from build123d import *

# Parameters (mm, degrees)
F0_R     = 26.85
F0_R_2   = 2.5
F1_DEPTH = 7
F2_SIZE  = 1.5
F3_SIZE  = 5


with BuildPart() as f1:
    # F0 (on Front) → F1 (new body)
    with BuildSketch(Plane.XZ):
        with Locations((0, 7)):
            Circle(F0_R)
        with Locations((-13.75, 0)):
            Circle(F0_R_2, mode=Mode.SUBTRACT)
        with Locations((0, -1)):
            Circle(F0_R_2, mode=Mode.SUBTRACT)
        with Locations((0, 7)):
            Circle(F0_R_2, mode=Mode.SUBTRACT)
        with Locations((13.75, 0)):
            Circle(F0_R_2, mode=Mode.SUBTRACT)
        with Locations((0, 15)):
            Circle(F0_R_2, mode=Mode.SUBTRACT)
    extrude(amount=F1_DEPTH)

    # F2
    f2_edges = [f1.edges().sort_by_distance(p)[0] for p in [
        (-16.25, -7, 0),
        (11.25, -7, 0),
    ]]
    chamfer(f2_edges, length=F2_SIZE)

    # F3
    f3_edges = [f1.edges().sort_by_distance(p)[0] for p in [
        (-26.85, -7, 7),
    ]]
    chamfer(f3_edges, length=F3_SIZE)


solid = f1.part
Model file for the job. Use its own axes, mm. Round coordinates to 2 decimals unless told otherwise and drop trailing zeros. Loops run counter-clockwise (first coordinate to the right, second up) from the corner with the lowest first, then second, coordinate; pieces in that order, holes last. Notation, with made-up numbers: (-18.75, -14) - (35.25, -14) arc R23 ccw to (35.25, 12) - close; hole circle Ø2 at (-12.5, -6.5). An arc over 180 degrees is marked (long way). Write each question's results on one line, items separated by ' | '.
(1) Saw through at C-C, the plane z = -1. Count the separate pieces of the cut face and the enclosed holes in it, then the cut area to 3 significant figures.
Answer below:
separate pieces: 4 | enclosed holes: 0 | area: 229 mm^2
(2) Saw through at B-B, the plane y = -4.5. List the corners of the cut face in (x, z), then the cut area to 3 significant figures.
Answer below:
outline: circle Ø48.7 at (0, 7); hole circle Ø5 at (-13.75, 0); hole circle Ø5 at (0, -1); hole circle Ø5 at (0, 7); hole circle Ø5 at (0, 15); hole circle Ø5 at (13.75, 0) | area: 1,760 mm^2
(3) Saw through at D-D, the plane y = -0.75. List the corners of the cut face in (x, z).
Answer below:
outline: circle Ø53.7 at (0, 7); hole circle Ø5 at (-13.75, 0); hole circle Ø5 at (0, -1); hole circle Ø5 at (0, 7); hole circle Ø5 at (0, 15); hole circle Ø5 at (13.75, 0)
(4) Mould opens along Z. For faces 1 (the flat face through (6, 0, 7)), 2 (the conical face through (-4.804, -6.687, -14.636)), 3 (the cylindrical face through (-0.54, -3.45, -3.44)) say: released by +Z, released by -Z, zero draft, split by the parting line, or undercut.
Answer below:
face 1: zero draft | face 2: split by the parting line | face 3: undercut
(5) Wall check: L1, parallel to Z at x = 0, y = -2.5; L2, parallel to Z at x = 0, y = -2.25; L3, parallel to X at y = -0.75, z = -1.5. Give the ranges that are in metal, low to high.
Answer below:
L1: z = -19.35 to -3.5, 1.5 to 4.5, 9.5 to 12.5, 17.5 to 33.35 | L2: z = -19.6 to -3.5, 1.5 to 4.5, 9.5 to 12.5, 17.5 to 33.6 | L3: x = -25.47 to -15.75, -11.75 to -2.45, 2.45 to 11.75, 15.75 to 25.47
(6) Pin check, flat tips, straight feed: pin 1 (4 mm diameter, centred on x = -9, z = 6, fed in from +Y); pin 2 (4.5 mm diameter, centred on x = -13.75, z = 0, fed in from -Y); pin 3 (1 mm diameter, centred on x = -4, y = -5, fed in from +Z); pin 4 (4 mm diameter, centred on y = -1.5, z = -14, fed in from +X). Stop position of each tip, or through.
Answer below:
pin 1: stops at y = 0 | pin 2: passes through | pin 3: stops at z = 31.03 | pin 4: stops at x = 18.97
(7) Saw through at A-A, the plane z = 7. List the corners of the cut face in (x, y), then the cut area to 3 significant figures.
Answer below:
outline: (-26.85, -2) - (-21.85, -7) - (-2.5, -7) - (-2.5, 0) - (-26.85, 0) - close; (2.5, -7) - (21.85, -7) - (26.85, -2) - (26.85, 0) - (2.5, 0) - close | area: 316 mm^2
